from build123d import *

# Parameters (mm, degrees)
SKETCH1_W           = 111.1
SKETCH1_H           = 121.6
BOSS_EXTRUDE1_DEPTH = 26.6
SKETCH2_W           = 104.5
SKETCH2_H           = 115
CUT_EXTRUDE1_DEPTH  = 26
SKETCH5_R           = 2.4
CUT_EXTRUDE3_DEPTH  = 4
SKETCH7_W           = 6.3
SKETCH7_H           = 3.8
SKETCH7_W_2         = 11
SKETCH7_H_2         = 7.6
CUT_EXTRUDE4_DEPTH  = 4
SKETCH8_W           = 117
SKETCH8_H           = 1.5
CUT_EXTRUDE5_DEPTH  = 110
SKETCH9_W           = 117
SKETCH9_H           = 0.5
CUT_EXTRUDE6_DEPTH  = 3.5


with BuildPart() as part:
    # Sketch1 → Boss-Extrude1 (new body)
    with BuildSketch(Plane(origin=(0, 0, 0), x_dir=(1, 0, 0), z_dir=(0, 1, 0))):
        Rectangle(SKETCH1_W, SKETCH1_H)
    extrude(amount=BOSS_EXTRUDE1_DEPTH)

    # Sketch2 → Cut-Extrude1 (cut)
    with BuildSketch(Plane(origin=(0, 26.6, 0), x_dir=(1, 0, 0), z_dir=(0, 1, 0))):
        Rectangle(SKETCH2_W, SKETCH2_H)
    extrude(amount=-CUT_EXTRUDE1_DEPTH, mode=Mode.SUBTRACT)

    # Sketch5 → Cut-Extrude3 (cut)
    with BuildSketch(Plane(origin=(0, 0, -60.8), x_dir=(-1, 0, 0), z_dir=(0, 0, -1))):
        with Locations((42.85, 10.7)):
            Circle(SKETCH5_R)
        with Locations((4.45, 10.7)):
            Circle(SKETCH5_R)
        Polygon((9.45, 2.3), (37.85, 2.3), (37.85, 15.816960095), (33.1, 20.566960095), (14.2, 20.566960095), (9.45, 15.816960095), align=None)
    extrude(amount=-CUT_EXTRUDE3_DEPTH, mode=Mode.SUBTRACT)

    # Sketch7 → Cut-Extrude4 (cut)
    with BuildSketch(Plane.XY.offset(60.8)):
        with Locations((47.4, 3.9)):
            Rectangle(SKETCH7_W, SKETCH7_H)
        with Locations((37.4, 3.9)):
            Rectangle(SKETCH7_W, SKETCH7_H)
        with Locations((27.4, 3.9)):
            Rectangle(SKETCH7_W, SKETCH7_H)
        with Locations((-1.95, 5.8)):
            Rectangle(SKETCH7_W_2, SKETCH7_H_2)
    extrude(amount=-CUT_EXTRUDE4_DEPTH, mode=Mode.SUBTRACT)

    # Sketch8 → Cut-Extrude5 (cut)
    with BuildSketch(Plane(origin=(55.55, 0, 0), x_dir=(0, 0, -1), z_dir=(1, 0, 0))):
        with Locations((-0.072921922, 25.35)):
            Rectangle(SKETCH8_W, SKETCH8_H)
    extrude(amount=-CUT_EXTRUDE5_DEPTH, mode=Mode.SUBTRACT)

    # Sketch9 → Cut-Extrude6 (cut)
    with BuildSketch(Plane(origin=(55.55, 0, 0), x_dir=(0, 0, -1), z_dir=(1, 0, 0))):
        with Locations((-0.072921922, 26.35)):
            Rectangle(SKETCH9_W, SKETCH9_H)
    extrude(amount=-CUT_EXTRUDE6_DEPTH, mode=Mode.SUBTRACT)


solid = part.part
Can you work these out from the model? Positions are in its coordinate system, mm. A direction names the side the tool comes from. Coordinates: 2 decimals unless noted, no trailing zeros. Loops run counter-clockwise (first coordinate to the right, second up) from the corner with the lowest first, then second, coordinate; pieces in that order, holes last. Notation, with made-up numbers: M -5,4 L 20,4 A22 ccw 20,34 Z; hole C 1,72.5 d1. An arc over 180 degrees is marked long. Return JSON: item names as keys, results as strings. Group by question number.
Item 1: I'm going to push flat-ended pins straight in: pin 1 Ø4 at (x, z) = (-32.5, 21) entering from +Y; pin 2 Ø3 at (x, y) = (-25, 11) entering from -Z. Where does each tip first touch, or does it pass through?
Item 2: Thinking about a two-plate mould opening in Y: for faces 1 (the flat face through (55.55, 10, 1)), 2 (the flat face through (-1, 0, -1)), 3 (the flat face through (-2, 9.6, 59)), 4 (the flat face through (-35.508, 18.159, -59.173)), which applies, released by +Y, released by -Y, zero draft, split by the parting line, or undercut?
Item 3: Imagine slicing it at D-D (x = 18). Please give me the cut outline in (y, z), and give its area (3 significant figures).
Item 4: Imagine slicing it at A-A (x = -42.85). Please give me the cut outline in (y, z), and give its area (3 significant figures).
Item 5: Imagine slicing it at C-C (z = 51). Please give me the cut outline in (x, y).
Item 6: If I drill on L1, parallel to X at y = 9, z = -31; L2, parallel to Z at x = 25, y = 10.5; L3, parallel to Z at x = -11.5, y = 11, over which ranges is the centre line in solid material (lowest first)? Write a range as from..to.
Item 7: Imagine slicing it at B-B (x = -4.45). Please give me the cut outline in (y, z).
Item 8: On a 3-axis mill with a long thin cutter (end or side, diameter ignored), from which of +Z, -Z, +X, -X, +Y, -Y can I reach the whole of each face in a straight line? I mean faces 5 (the flat face through (44.25, 4, 59)), 6 (the cylindrical face through (-2.545, 9.24, -59.173)), 7 (the flat face through (-55.55, 13, 1)). Say none if no direction works.
Verdict:
{
 "1": {"pin 1": "stops at y = 0.6", "pin 2": "stops at z = 57.5"},
 "2": {"face 1": "zero draft", "face 2": "released by -Y", "face 3": "undercut", "face 4": "undercut"},
 "3": {"outline": "M 0,-60.8 L 26.6,-60.8 L 26.6,-57.5 L 26.1,-57.5 L 26.1,-58.43 L 24.6,-58.43 L 24.6,-57.5 L 0.6,-57.5 L 0.6,57.5 L 24.6,57.5 L 24.6,58.57 L 26.1,58.57 L 26.1,57.5 L 26.6,57.5 L 26.6,60.8 L 0,60.8 Z", "area": "242 mm^2"},
 "4": {"outline": "M 0,-60.8 L 8.3,-60.8 L 8.3,-57.5 L 0.6,-57.5 L 0.6,57.5 L 24.6,57.5 L 24.6,58.57 L 26.1,58.57 L 26.1,57.5 L 26.6,57.5 L 26.6,60.8 L 0,60.8 Z; M 13.1,-60.8 L 26.6,-60.8 L 26.6,-57.5 L 26.1,-57.5 L 26.1,-58.43 L 24.6,-58.43 L 24.6,-57.5 L 13.1,-57.5 Z", "area": "226 mm^2"},
 "5": {"outline": "M -55.55,0 L 55.55,0 L 55.55,24.6 L 52.25,24.6 L 52.25,0.6 L -52.25,0.6 L -52.25,24.6 L -54.45,24.6 L -54.45,26.1 L -52.25,26.1 L -52.25,26.6 L -55.55,26.6 Z"},
 "6": {"L1": "x = -55.55..-52.25, 52.25..55.55", "L2": "z = -60.8..-57.5, 57.5..60.8", "L3": "z = 57.5..60.8"},
 "7": {"outline": "M 0,-60.8 L 8.3,-60.8 L 8.3,-57.5 L 0.6,-57.5 L 0.6,57.5 L 2,57.5 L 2,60.8 L 0,60.8 Z; M 9.6,57.5 L 24.6,57.5 L 24.6,58.57 L 26.1,58.57 L 26.1,57.5 L 26.6,57.5 L 26.6,60.8 L 9.6,60.8 Z; M 13.1,-60.8 L 26.6,-60.8 L 26.6,-57.5 L 26.1,-57.5 L 26.1,-58.43 L 24.6,-58.43 L 24.6,-57.5 L 13.1,-57.5 Z"},
 "8": {"face 5": "+Z", "face 6": "-Z", "face 7": "+Z, -Z, -X, +Y, -Y"}
}
